from build123d import *

# Parameters (mm, degrees)
F0_W           = 13
F0_H           = 40
F0_W_2         = 24
F1_DEPTH       = 19
F3_DEPTH       = 50
F4_DEPTH       = 12
F6_D           = 5
F8_D           = 3
F8_CBORE_D     = 6
F8_CBORE_DEPTH = 7
F9_R           = 1.5
F10_DEPTH      = 3


with BuildPart() as f1:
    # F0 (on Top) → F1 (new body)
    with BuildSketch(Plane.XY):
        with Locations((-43.5, -20)):
            Rectangle(F0_W, F0_H)
        with Locations((-25, -20)):
            Rectangle(F0_W_2, F0_H)
        with Locations((-6.5, -20)):
            Rectangle(F0_W, F0_H)
    extrude(amount=F1_DEPTH)

    # F2 (on face) → F3 (cut)
    with BuildSketch(Plane.YZ):
        with BuildLine():
            Line((-14.0839202169, 19), (-25.9160797831, 19))
            ThreePointArc((-25.9160797831, 19), (-20, 14), (-14.0839202169, 19))
        make_face()
    extrude(amount=-F3_DEPTH, mode=Mode.SUBTRACT)

    # F0 (on Top) → F4 (join)
    with BuildSketch(Plane.XY):
        with Locations((-6.5, -20)):
            Rectangle(F0_W, F0_H)
        with Locations((-43.5, -20)):
            Rectangle(F0_W, F0_H)
    extrude(amount=-F4_DEPTH)

    # F6 (through all)
    with Locations(Plane.XY.offset(19)):
        with Locations((-6.5, -32), (-43.5, -32), (-43.5, -8), (-6.5, -8)):
            Hole(F6_D / 2)

    # F8 (through all)
    with Locations(Plane.XY.offset(19)):
        with Locations((-25, -10), (-25, -30)):
            CounterBoreHole(F8_D / 2, F8_CBORE_D / 2, F8_CBORE_DEPTH)

    # F9 (on face) → F10 (cut)
    with BuildSketch(Plane(origin=(0, 0, 0), x_dir=(1, 0, 0), z_dir=(0, 0, -1))):
        Polygon((-23.2679491924, 13), (-26.7320508076, 13), (-28.4641016151, 10), (-26.7320508076, 7), (-23.2679491924, 7), (-21.5358983849, 10), align=None)
        with Locations((-25, 10)):
            Circle(F9_R, mode=Mode.SUBTRACT)
        Polygon((-23.2679491924, 33), (-26.7320508076, 33), (-28.4641016151, 30), (-26.7320508076, 27), (-23.2679491924, 27), (-21.5358983849, 30), align=None)
        with Locations((-25, 30)):
            Circle(F9_R, mode=Mode.SUBTRACT)
    extrude(amount=-F10_DEPTH, mode=Mode.SUBTRACT)


solid = f1.part
Input: part model. Units: mm. Frame: model coordinates. A direction names the side the tool comes from. Give positions to 0.01 mm unless a question says otherwise; leave off trailing zeros. Write each loop counter-clockwise with the first axis right and the second up, starting at its lowest first coordinate (ties: lowest second). Pieces come first, ordered by that corner, then holes. Notation, with made-up numbers: (35.5, -31.5) -> (71.5, -31.5) arc R16 cw to (71.5, -25.5) -> close; hole circle Ø5 at (79, 10). An arc over 180 degrees is marked (long way). Use one line per item in the form item = value. Start each with the question number.
1) Section query A-A on x = -6.5. Return the cut outline in (y, z).
2) Section query B-B on z = 9.5. Return the cut outline in (x, y).
3) Draft query along Y for faces 1 (the flat face through (-23.5, -10.7, 3)), 2 (the flat face through (-25, 0, 7)), 3 (the flat face through (-25, -20, 0)), 4 (the flat face through (-25, -40, 7)). Return one class per face: pulls with the +Y half, pulls with the -Y half, needs draft (parallel to the pull), parting line crosses it, or undercut.
4) Set-up query: faces 5 (the cylindrical face through (-28, -10, 16)), 6 (the flat face through (-27.6, -11.5, 1.5)), 7 (the cylindrical face through (-25, -20, 14)). Return all of +Z, -Z, +X, -X, +Y, -Y with unobstructed straight access to the full face (end or side cutting, diameter ignored); none if empty.
5) Section query D-D on x = -20. Return the cut outline in (y, z).
6) Ray query, probe 1 along Y at (x, z) = (-43.5, 9); probe 2 along Y at (x, z) = (-25, 2); probe 3 along X at (y, z) = (-12, -0.5). Return the intervals inside material, ascending. Write a range as from..to.
7) Pin query (flat end, axial travel): pin 1 (9.5 mm diameter, centred on x = -25, y = -30, fed in from -Z); pin 2 (1.8 mm diameter, centred on x = -25.5, y = -29, fed in from -Z); pin 3 (5 mm diameter, centred on x = -25, y = -10, fed in from +Z). Return the tip coordinate at first contact, or that it passes through.
8) Section query C-C on y = -4.5. Return the cut outline in (x, z).
Outcome:
q1.outline = (-40, -12) -> (-34.5, -12) -> (-34.5, 19) -> (-40, 19) -> close; (-29.5, -12) -> (-10.5, -12) -> (-10.5, 19) -> (-14.08, 19) arc R6 cw to (-25.92, 19) -> (-29.5, 19) -> close; (-5.5, -12) -> (0, -12) -> (0, 19) -> (-5.5, 19) -> close
q2.outline = (-50, -40) -> (0, -40) -> (0, 0) -> (-50, 0) -> close; hole circle Ø5 at (-43.5, -32); hole circle Ø5 at (-43.5, -8); hole circle Ø3 at (-25, -30); hole circle Ø3 at (-25, -10); hole circle Ø5 at (-6.5, -32); hole circle Ø5 at (-6.5, -8)
q3.face_1 = undercut
q3.face_2 = pulls with the +Y half
q3.face_3 = needs draft
q3.face_4 = pulls with the -Y half
q4.face_5 = +Z
q4.face_6 = -Z
q4.face_7 = +Z, +X, -X
q5.outline = (-40, 0) -> (0, 0) -> (0, 19) -> (-14.08, 19) arc R6 cw to (-25.92, 19) -> (-40, 19) -> close
q6.probe_1 = -40..-34.5, -29.5..-10.5, -5.5..0
q6.probe_2 = -40..-33, -27..-13, -7..0
q6.probe_3 = -50..-37, -13..0
q7.pin_1 = 0
q7.pin_2 = 3
q7.pin_3 = 12
q8.outline = (-50, -12) -> (-37, -12) -> (-37, 0) -> (-13, 0) -> (-13, -12) -> (0, -12) -> (0, 19) -> (-50, 19) -> close
